Work out the finished part from the listing and answer in its coordinate system (mm). Face numbers are marked on the shaded views. A direction names the side the tool comes from. Round coordinates to 2 decimals unless told otherwise and drop trailing zeros. Write each loop counter-clockwise with the first axis right and the second up, starting at its lowest first coordinate (ties: lowest second). Pieces come first, ordered by that corner, then holes. Notation, with made-up numbers: M 71.25,9 L 127.25,9 A19 ccw 127.25,20 Z; hole C -3,-40 d11. An arc over 180 degrees is marked long. Answer in a Markdown table with one row per item.
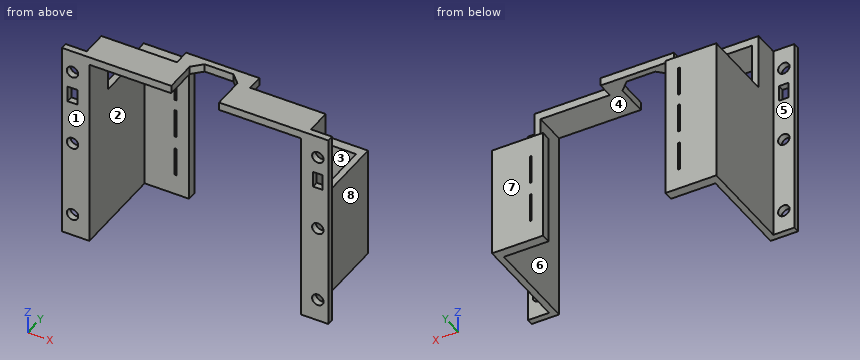
```python
from build123d import *

# Parameters (mm, degrees)
SKETCH1_W            = 70.4
SKETCH1_H            = 2
BOSS_EXTRUDE2_DEPTH  = 10
SKETCH2_W            = 2
SKETCH2_H            = 55
BOSS_EXTRUDE3_DEPTH  = 10
SKETCH3_W            = 19
SKETCH3_H            = 3
BOSS_EXTRUDE4_DEPTH  = 2
SKETCH4_W            = 15
SKETCH4_H            = 10
CUT_EXTRUDE2_DEPTH   = 2
SKETCH5_W            = 2
SKETCH5_H            = 3
BOSS_EXTRUDE5_DEPTH  = 1
SKETCH6_W            = 2
SKETCH6_H            = 3
BOSS_EXTRUDE6_DEPTH  = 1
SKETCH7_W            = 57
SKETCH7_H            = 2
BOSS_EXTRUDE7_DEPTH  = 6.6
SKETCH8_W            = 57
SKETCH8_H            = 2
BOSS_EXTRUDE8_DEPTH  = 6.6
BOSS_EXTRUDE9_DEPTH  = 5
SKETCH12_W           = 2
SKETCH12_H           = 5
SKETCH12_H_2         = 40
SKETCH12_H_3         = 30
BOSS_EXTRUDE10_DEPTH = 20
BOSS_EXTRUDE11_DEPTH = 3
SKETCH14_W           = 0.5
SKETCH14_H           = 9
CUT_EXTRUDE3_DEPTH   = 3
SKETCH15_W           = 38.4
SKETCH15_H           = 45
CUT_EXTRUDE4_DEPTH   = 3
BOSS_EXTRUDE12_DEPTH = 0.5
SKETCH17_R           = 1.8
SKETCH17_W           = 3
SKETCH17_H           = 5
CUT_EXTRUDE6_DEPTH   = 3
SKETCH18_W           = 2.5
SKETCH18_H           = 3
BOSS_EXTRUDE13_DEPTH = 1
SKETCH19_W           = 2.5
SKETCH19_H           = 3
BOSS_EXTRUDE14_DEPTH = 1
SKETCH20_W           = 23
SKETCH20_H           = 2.5
BOSS_EXTRUDE15_DEPTH = 2
CUT_EXTRUDE8_DEPTH   = 3


with BuildPart() as part:
    # Sketch1 → Boss-Extrude2 (new body)
    with BuildSketch(Plane(origin=(0, 0, 0), x_dir=(1, 0, 0), z_dir=(0, 1, 0))):
        with Locations((35.2, 1)):
            Rectangle(SKETCH1_W, SKETCH1_H)
    extrude(amount=BOSS_EXTRUDE2_DEPTH)

    # Sketch2 → Boss-Extrude3 (add)
    with BuildSketch(Plane(origin=(0, 10, 0), x_dir=(1, 0, 0), z_dir=(0, 1, 0))):
        with Locations((1, 29.5)):
            Rectangle(SKETCH2_W, SKETCH2_H)
        with Locations((69.4, 29.5)):
            Rectangle(SKETCH2_W, SKETCH2_H)
    extrude(amount=-BOSS_EXTRUDE3_DEPTH)

    # Sketch3 → Boss-Extrude4 (add)
    with BuildSketch(Plane.XY):
        with Locations((35.2, 11.5)):
            Rectangle(SKETCH3_W, SKETCH3_H)
    extrude(amount=-BOSS_EXTRUDE4_DEPTH)

    # Sketch4 → Cut-Extrude2 (cut)
    with BuildSketch(Plane.XY):
        with Locations((35.2, 5)):
            Rectangle(SKETCH4_W, SKETCH4_H)
    extrude(amount=-CUT_EXTRUDE2_DEPTH, mode=Mode.SUBTRACT)

    # Sketch5 → Boss-Extrude5 (add)
    with BuildSketch(Plane.ZY.offset(-25.7)):
        with Locations((-1, 11.5)):
            Rectangle(SKETCH5_W, SKETCH5_H)
    extrude(amount=BOSS_EXTRUDE5_DEPTH)

    # Sketch6 → Boss-Extrude6 (add)
    with BuildSketch(Plane(origin=(44.7, 0, 0), x_dir=(0, 0, -1), z_dir=(1, 0, 0))):
        with Locations((1, 11.5)):
            Rectangle(SKETCH6_W, SKETCH6_H)
    extrude(amount=BOSS_EXTRUDE6_DEPTH)

    # Sketch7 → Boss-Extrude7 (add)
    with BuildSketch(Plane.ZY):
        with Locations((-28.5, 1)):
            Rectangle(SKETCH7_W, SKETCH7_H)
    extrude(amount=BOSS_EXTRUDE7_DEPTH)

    # Sketch8 → Boss-Extrude8 (add)
    with BuildSketch(Plane(origin=(70.4, 0, 0), x_dir=(0, 0, -1), z_dir=(1, 0, 0))):
        with Locations((28.5, 1)):
            Rectangle(SKETCH8_W, SKETCH8_H)
    extrude(amount=BOSS_EXTRUDE8_DEPTH)

    # Sketch10 → Boss-Extrude9 (add)
    with BuildSketch(Plane(origin=(0, 0, -57), x_dir=(-1, 0, 0), z_dir=(0, 0, -1))):
        Polygon((-2, 10), (-2, 0), (6.6, 0), (6.6, 2), (0, 2), (0, 10), align=None)
        Polygon((-77, 0), (-68.4, 0), (-68.4, 10), (-70.4, 10), (-70.4, 2), (-77, 2), align=None)
    extrude(amount=BOSS_EXTRUDE9_DEPTH)

    # Sketch12 → Boss-Extrude10 (add)
    with BuildSketch(Plane(origin=(0, 10, 0), x_dir=(1, 0, 0), z_dir=(0, 1, 0))):
        with Locations((1, 59.5)):
            Rectangle(SKETCH12_W, SKETCH12_H)
        with Locations((1, 37)):
            Rectangle(SKETCH12_W, SKETCH12_H_2)
        with Locations((69.4, 42)):
            Rectangle(SKETCH12_W, SKETCH12_H_3)
        with Locations((69.4, 59.5)):
            Rectangle(SKETCH12_W, SKETCH12_H)
    extrude(amount=BOSS_EXTRUDE10_DEPTH)

    # Sketch13 → Boss-Extrude11 (add)
    with BuildSketch(Plane(origin=(0, 30, 0), x_dir=(1, 0, 0), z_dir=(0, 1, 0))):
        Polygon((0, 17), (35.2, 17), (35.2, 27), (70.4, 27), (70.4, 62), (0, 62), align=None)
    extrude(amount=BOSS_EXTRUDE11_DEPTH)

    # Sketch14 → Cut-Extrude3 (cut)
    with BuildSketch(Plane(origin=(0, 33, 0), x_dir=(1, 0, 0), z_dir=(0, 1, 0))):
        with Locations((11.7, 51)):
            Rectangle(SKETCH14_W, SKETCH14_H)
        with Locations((11.7, 38)):
            Rectangle(SKETCH14_W, SKETCH14_H)
        with Locations((11.7, 25.5)):
            Rectangle(SKETCH14_W, SKETCH14_H)
        with Locations((58.2, 51)):
            Rectangle(SKETCH14_W, SKETCH14_H)
        with Locations((58.2, 38)):
            Rectangle(SKETCH14_W, SKETCH14_H)
    extrude(amount=-CUT_EXTRUDE3_DEPTH, mode=Mode.SUBTRACT)

    # Sketch15 → Cut-Extrude4 (cut)
    with BuildSketch(Plane(origin=(0, 33, 0), x_dir=(1, 0, 0), z_dir=(0, 1, 0))):
        with Locations((35.2, 39.5)):
            Rectangle(SKETCH15_W, SKETCH15_H)
    extrude(amount=-CUT_EXTRUDE4_DEPTH, mode=Mode.SUBTRACT)

    # Sketch16 → Boss-Extrude12 (add)
    with BuildSketch(Plane.XY):
        Polygon((-6.6, 0), (27.7, 0), (27.7, 10), (42.7, 10), (42.7, 0), (77, 0), (77, 2), (70.4, 2), (70.4, 10), (45.7, 10), (45.7, 13), (24.7, 13), (24.7, 10), (0, 10), (0, 2), (-6.6, 2), align=None)
    extrude(amount=BOSS_EXTRUDE12_DEPTH)

    # Sketch17 → Cut-Extrude6 (cut)
    with BuildSketch(Plane(origin=(0, 2, 0), x_dir=(1, 0, 0), z_dir=(0, 1, 0))):
        with Locations(Location((-3.3, 55, 0), (0, 0, 270))):
            Circle(SKETCH17_R)
        with Locations(Location((73.7, 55, 0), (0, 0, 270))):
            Circle(SKETCH17_R)
        with Locations(Location((-3.3, 6.5, 0), (0, 0, 270))):
            Circle(SKETCH17_R)
        with Locations(Location((73.7, 6.5, 0), (0, 0, 270))):
            Circle(SKETCH17_R)
        with Locations(Location((-3.3, 30.75, 0), (0, 0, 270))):
            Circle(SKETCH17_R)
        with Locations(Location((73.7, 30.75, 0), (0, 0, 270))):
            Circle(SKETCH17_R)
        with Locations((-3.3, 14.5)):
            Rectangle(SKETCH17_W, SKETCH17_H)
        with Locations((73.7, 14.5)):
            Rectangle(SKETCH17_W, SKETCH17_H)
    extrude(amount=-CUT_EXTRUDE6_DEPTH, mode=Mode.SUBTRACT)

    # Sketch18 → Boss-Extrude13 (add)
    with BuildSketch(Plane.ZY.offset(-24.7)):
        with Locations((-0.75, 11.5)):
            Rectangle(SKETCH18_W, SKETCH18_H)
    extrude(amount=BOSS_EXTRUDE13_DEPTH)

    # Sketch19 → Boss-Extrude14 (add)
    with BuildSketch(Plane(origin=(45.7, 0, 0), x_dir=(0, 0, -1), z_dir=(1, 0, 0))):
        with Locations((0.75, 11.5)):
            Rectangle(SKETCH19_W, SKETCH19_H)
    extrude(amount=BOSS_EXTRUDE14_DEPTH)

    # Sketch20 → Boss-Extrude15 (add)
    with BuildSketch(Plane(origin=(0, 13, 0), x_dir=(1, 0, 0), z_dir=(0, 1, 0))):
        with Locations((35.2, 0.75)):
            Rectangle(SKETCH20_W, SKETCH20_H)
    extrude(amount=BOSS_EXTRUDE15_DEPTH)

    # Sketch21 → Cut-Extrude8 (cut)
    with BuildSketch(Plane.XY.offset(0.5)):
        Polygon((27.7, 10), (30.7, 13), (39.7, 13), (42.7, 10), align=None)
    extrude(amount=-CUT_EXTRUDE8_DEPTH, mode=Mode.SUBTRACT)


solid = part.part
```
1. Consider line 1 along X through (y, z) = (0.8, -6.5); line 2 along Z through (x, y) = (73.7, 1.3); line 3 along X through (y, z) = (5, -41.5). Determine where each line is inside the solid, lowest interval first. Write a range as from..to.
Calculated:
| item | result |
|---|---|
| line 1 | x = -6.6..-5.1, -1.5..2, 68.4..71.9, 75.5..77 |
| line 2 | z = -62..-56.8, -53.2..-32.55, -28.95..-17, -12..-8.3, -4.7..0.5 |
| line 3 | x = 0..2, 68.4..70.4 |
2. Determine the mould class of the marked faces 6, 7 and 8 for opening direction X: released by +X, released by -X, zero draft, split by the parting line, or undercut.
Calculated:
| item | result |
|---|---|
| face 6 | undercut |
| face 7 | zero draft |
| face 8 | released by +X |
3. Given pin 1 (3 mm diameter, centred on x = -3.3, z = -55, fed in from -Y); pin 2 (5 mm diameter, centred on x = 54.5, y = 7, fed in from -Z); pin 3 (3.5 mm diameter, centred on y = 31.5, z = -50.5, fed in from -X); pin 4 (0.8 mm diameter, centred on y = 12, z = -1, fed in from -X), each flat-ended and moving along its own axis, determine where each tip first touches the part or whether it passes through.
Calculated:
| item | result |
|---|---|
| pin 1 | passes through |
| pin 2 | stops at z = -2 |
| pin 3 | stops at x = 0 |
| pin 4 | stops at x = 23.7 |
4. A tool of negligible diameter and unlimited length cuts with its end or side. For the marked faces 1, 2, 3, 4 and 5, from which of +Z, -Z, +X, -X, +Y, -Y can it reach the whole face along a straight path? Write none if from no direction.
Calculated:
| item | result |
|---|---|
| face 1 | +Z, -Z, +X, -X, -Y |
| face 2 | -Z, -Y |
| face 3 | +Z, -Z, -Y |
| face 4 | -Z, +Y, -Y |
| face 5 | +Z, -Z, -X, +Y |
5. The part is cut by section B-B (y = 24.5). Determine the outline of the cut face in (x, z).
Calculated:
| item | result |
|---|---|
| outline | M 0,-62 L 2,-62 L 2,-17 L 0,-17 Z; M 68.4,-62 L 70.4,-62 L 70.4,-27 L 68.4,-27 Z |
6. The part is cut by section C-C (z = -58). Determine the outline of the cut face in (x, y), plus the area to 3 significant figures.
Calculated:
| item | result |
|---|---|
| outline | M -6.6,0 L 2,0 L 2,30 L 16,30 L 16,33 L 0,33 L 0,2 L -6.6,2 Z; M 54.4,30 L 68.4,30 L 68.4,0 L 77,0 L 77,2 L 70.4,2 L 70.4,33 L 54.4,33 Z |
| area | 242 mm² |
7. The part is cut by section D-D (y = 11). Determine the outline of the cut face in (x, z), plus the area to 3 significant figures.
Calculated:
| item | result |
|---|---|
| outline | M 0,-62 L 2,-62 L 2,-17 L 0,-17 Z; M 23.7,-2 L 28.7,-2 L 28.7,0.5 L 23.7,0.5 Z; M 41.7,-2 L 46.7,-2 L 46.7,0.5 L 41.7,0.5 Z; M 68.4,-62 L 70.4,-62 L 70.4,-27 L 68.4,-27 Z |
| area | 185 mm² |
8. The part is cut by section A-A (x = 6). Determine the outline of the cut face in (y, z).
Calculated:
| item | result |
|---|---|
| outline | M 0,-2 L 10,-2 L 10,0.5 L 0,0.5 Z; M 30,-62 L 33,-62 L 33,-17 L 30,-17 Z |
